For this review, take the finished solid that the model builds, in its own axes (mm). A direction names the side the tool comes from. Give positions to 0.01 mm unless a question says otherwise; leave off trailing zeros. Order: outer loops, then holes, each group sorted by start corner. A loop starts at its lowest first (then second) coordinate and runs counter-clockwise, first axis right, second up. Notation, with made-up numbers: (3, 40.25) -> (17, 40.25) arc R18 ccw to (17, 72.25) -> close; hole circle Ø6 at (31.5, 2). An arc over 180 degrees is marked (long way). Return JSON: item names as keys, results as strings. Group by question number.
1) The part is to be moulded in two halves that separate along Y. For faces 1 (the face through (12, -1, 0)), 2 (the face through (0, -54.837, 9)), 3 (the face through (11, -1, 2.54)), say which applies: released by +Y, released by -Y, zero draft, split by the parting line, or undercut.
2) Add section D-D (x = 12.5). Give the boundary of the cut face in (y, z).
3) Add section C-C (y = -35.5). Give the boundary of the cut face in (x, z).
4) To check wall thickness, follow line 1 along Y through (x, z) = (-0.5, 10.5); line 2 along X through (y, z) = (-16, 8.75); line 3 along Y through (x, z) = (0, 1.25). State the ranges of each line that lie inside material, in increasing order.
5) For faces 4 (the face through (51.15, -53.73, 9.39)), 5 (the face through (0, 49.272, 10)), list the 3-axis set-ups (+Z, -Z, +X, -X, +Y, -Y) from which the entire face can be reached by the end or side of a thin tool; tool diameter is ignored.
6) Add section A-A (x = 0). Give the boundary of the cut face in (y, z), then the cut area to 3 significant figures.
7) Add section B-B (y = 0). Give the boundary of the cut face in (x, z).
8) Insertion check: P1, Ø10, axis at x = 28.5, y = 29, coming from the +Z side. The pin has a flat end and moves straight along its axis. Give the tip position at first contact, or say it passes through.
from build123d import *

# Parameters (mm, degrees)
F0_W     = 106.68
F0_H     = 106.68
F0_W_2   = 101.6
F0_H_2   = 101.6
F1_DEPTH = 19.05
F2_W     = 104.656483978
F2_H     = 104.4136583805
F3_DEPTH = 2.54
F4_R     = 3.81
F5_DEPTH = 12.7
F6_SIZE  = 7.62
F7_R     = 1.27
F8_DEPTH = 38.1
F9_SIZE  = 0.508
F10_SIZE = 0.762
F11_SIZE = 0.762


with BuildPart() as f1:
    # F0 (on Top) → F1 (new body)
    with BuildSketch(Plane.XY):
        with Locations((0.6475270653, -1.4974073434)):
            Rectangle(F0_W, F0_H)
        with Locations((0.5357495129, -1.5282401264)):
            Rectangle(F0_W_2, F0_H_2, mode=Mode.SUBTRACT)
    extrude(amount=F1_DEPTH)

    # F2 (on Top) → F3 (join)
    with BuildSketch(Plane.XY):
        with Locations((0.6070565432, -1.821167767)):
            Rectangle(F2_W, F2_H)
    extrude(amount=F3_DEPTH)

    # F4 (on Top) → F5 (cut, symmetric)
    with BuildSketch(Plane.XY):
        Circle(F4_R)
    extrude(amount=F5_DEPTH, both=True, mode=Mode.SUBTRACT)

    # F6
    f6_edges = [f1.edges().sort_by_distance(p)[0] for p in [
        (-50.26425, 49.27176, 10.795),
        (51.33575, 49.27176, 10.795),
        (51.33575, -52.32824, 10.795),
        (-50.26425, -52.32824, 10.795),
    ]]
    chamfer(f6_edges, length=F6_SIZE)

    # F7 (on Top) → F8 (cut, symmetric)
    with BuildSketch(Plane.XY):
        with Locations((-50.1719862223, 49.0566454828)):
            Circle(F7_R)
        with Locations((51.3518936932, 49.0713790059)):
            Circle(F7_R)
        with Locations((51.4260791242, -52.4884499609)):
            Circle(F7_R)
        with Locations((-50.0576607883, -52.597168833)):
            Circle(F7_R)
    extrude(amount=F8_DEPTH, both=True, mode=Mode.SUBTRACT)

    # F9
    f9_edges = [f1.edges().sort_by_distance(p)[0] for p in [
        (-3.81, 0, 2.54),
        (-3.81, 0, 0),
    ]]
    chamfer(f9_edges, length=F9_SIZE)

    # F10
    f10_edges = [f1.edges().sort_by_distance(p)[0] for p in [
        (0.647527, -54.837407, 19.05),
        (-52.692473, -1.497407, 19.05),
        (53.987527, -1.497407, 19.05),
        (0.647527, 51.842593, 19.05),
        (51.33575, -1.52824, 19.05),
        (47.52575, -48.51824, 19.05),
        (0.53575, -52.32824, 19.05),
        (47.52575, 45.46176, 19.05),
        (0.53575, 49.27176, 19.05),
        (-46.45425, 45.46176, 19.05),
        (-50.26425, -1.52824, 19.05),
        (-46.45425, -48.51824, 19.05),
    ]]
    chamfer(f10_edges, length=F10_SIZE)

    # F11
    f11_edges = [f1.edges().sort_by_distance(p)[0] for p in [
        (-52.692473, -1.497407, 0),
        (0.647527, 51.842593, 0),
        (0.647527, -54.837407, 0),
        (53.987527, -1.497407, 0),
    ]]
    chamfer(f11_edges, length=F11_SIZE)


solid = f1.part
Evaluation:
{
 "1": {"face 1": "zero draft", "face 2": "released by -Y", "face 3": "undercut"},
 "2": {"outline": "(-54.84, 0.76) -> (-54.08, 0) -> (51.08, 0) -> (51.84, 0.76) -> (51.84, 18.29) -> (51.08, 19.05) -> (50.03, 19.05) -> (49.27, 18.29) -> (49.27, 2.54) -> (-52.33, 2.54) -> (-52.33, 18.29) -> (-53.09, 19.05) -> (-54.08, 19.05) -> (-54.84, 18.29) -> close"},
 "3": {"outline": "(-52.69, 0.76) -> (-51.93, 0) -> (53.23, 0) -> (53.99, 0.76) -> (53.99, 18.29) -> (53.23, 19.05) -> (52.1, 19.05) -> (51.34, 18.29) -> (51.34, 2.54) -> (-50.26, 2.54) -> (-50.26, 18.29) -> (-51.03, 19.05) -> (-51.93, 19.05) -> (-52.69, 18.29) -> close"},
 "4": {"line 1": "-54.84 to -52.33, 49.27 to 51.84", "line 2": "-52.69 to -50.26, 51.34 to 53.99", "line 3": "-54.84 to -3.81, 3.81 to 51.84"},
 "5": {"face 4": "+Z, -Z", "face 5": "+Z"},
 "6": {"outline": "(-54.84, 0.76) -> (-54.08, 0) -> (-4.32, 0) -> (-3.81, 0.51) -> (-3.81, 2.03) -> (-4.32, 2.54) -> (-52.33, 2.54) -> (-52.33, 18.29) -> (-53.09, 19.05) -> (-54.08, 19.05) -> (-54.84, 18.29) -> close; (3.81, 0.51) -> (4.32, 0) -> (51.08, 0) -> (51.84, 0.76) -> (51.84, 18.29) -> (51.08, 19.05) -> (50.03, 19.05) -> (49.27, 18.29) -> (49.27, 2.54) -> (4.32, 2.54) -> (3.81, 2.03) -> close", "area": "333 mm^2"},
 "7": {"outline": "(-52.69, 0.76) -> (-51.93, 0) -> (-4.32, 0) -> (-3.81, 0.51) -> (-3.81, 2.03) -> (-4.32, 2.54) -> (-50.26, 2.54) -> (-50.26, 18.29) -> (-51.03, 19.05) -> (-51.93, 19.05) -> (-52.69, 18.29) -> close; (3.81, 0.51) -> (4.32, 0) -> (53.23, 0) -> (53.99, 0.76) -> (53.99, 18.29) -> (53.23, 19.05) -> (52.1, 19.05) -> (51.34, 18.29) -> (51.34, 2.54) -> (4.32, 2.54) -> (3.81, 2.03) -> close"},
 "8": {"P1": "z = 2.54"}
}
